from build123d import *

# Parameters (mm, degrees)
SKETCH1_W           = 220
SKETCH1_H           = 40
BOSS_EXTRUDE1_DEPTH = 30
SKETCH2_R           = 10
CUT_EXTRUDE1_DEPTH  = 7
CUT_EXTRUDE2_START  = -30
SKETCH3_R           = 7
CUT_EXTRUDE2_DEPTH  = 23
SKETCH4_W           = 15
SKETCH4_H           = 40
CUT_EXTRUDE3_DEPTH  = 15
CUT_EXTRUDE4_START  = -30
SKETCH5_R           = 2.5
CUT_EXTRUDE4_DEPTH  = 15


with BuildPart() as part:
    # Sketch1 → Boss-Extrude1 (new body)
    with BuildSketch(Plane.XY):
        Rectangle(SKETCH1_W, SKETCH1_H)
    extrude(amount=BOSS_EXTRUDE1_DEPTH)

    # Sketch2 → Cut-Extrude1 (cut)
    with BuildSketch(Plane.XY):
        with Locations((90, 0)):
            Circle(SKETCH2_R)
    extrude(amount=CUT_EXTRUDE1_DEPTH, mode=Mode.SUBTRACT)

    # Sketch3 → Cut-Extrude2 (cut)
    with BuildSketch(Plane(origin=(0, 0, 0), x_dir=(-1, 0, 0), z_dir=(0, 0, -1)).offset(CUT_EXTRUDE2_START)):
        with Locations((-90, 0)):
            Circle(SKETCH3_R)
    extrude(amount=CUT_EXTRUDE2_DEPTH, mode=Mode.SUBTRACT)

    # Sketch4 → Cut-Extrude3 (cut)
    with BuildSketch(Plane(origin=(0, 0, 0), x_dir=(-1, 0, 0), z_dir=(0, 0, -1))):
        with Locations((-22.5, 0)):
            Rectangle(SKETCH4_W, SKETCH4_H)
        with Locations((2.5, 0)):
            Rectangle(SKETCH4_W, SKETCH4_H)
    extrude(amount=-CUT_EXTRUDE3_DEPTH, mode=Mode.SUBTRACT)

    # Sketch5 → Cut-Extrude4 (cut)
    with BuildSketch(Plane(origin=(0, 0, 0), x_dir=(-1, 0, 0), z_dir=(0, 0, -1)).offset(CUT_EXTRUDE4_START)):
        with Locations((-22.5, 10)):
            Circle(SKETCH5_R)
        with Locations((-22.5, -10)):
            Circle(SKETCH5_R)
        with Locations((2.5, -10)):
            Circle(SKETCH5_R)
        with Locations((2.5, 10)):
            Circle(SKETCH5_R)
    extrude(amount=CUT_EXTRUDE4_DEPTH, mode=Mode.SUBTRACT)


solid = part.part
Could you check a few things on this model? Use its own coordinates, in mm. A direction names the side the tool comes from. Give positions to 0.01 mm unless a question says otherwise; leave off trailing zeros. Order: outer loops, then holes, each group sorted by start corner. A loop starts at its lowest first (then second) coordinate and runs counter-clockwise, first axis right, second up. Notation, with made-up numbers: (89.25, -28.75) -> (124.25, -28.75) arc R19 cw to (124.25, 3.25) -> close; hole circle Ø2 at (-9, -39). An arc over 180 degrees is marked (long way). Answer in a Markdown table with one row per item. Add a question column.
Item 1: Please list where these lines run through material, in increasing order: probe 1 along X at (y, z) = (-12, 13.5); probe 2 along Y at (x, z) = (22.5, 24); probe 3 along X at (y, z) = (1.5, 6.75).
Item 2: I'm going to push flat-ended pins straight in: P1, Ø4, axis at x = -23.5, y = 14.5, coming from the -Z side; P2, Ø3, axis at x = -2.5, y = -10, coming from the -Z side; P3, Ø12, axis at x = 23, y = -2.5, coming from the -Z side; P4, Ø6, axis at x = 94.5, y = -4.5, coming from the -Z side. Where does each tip first touch, or does it pass through?
Item 3: Imagine slicing it at A-A (z = 3.5). List the corners of the cut face in (x, y) for me.
Item 4: Imagine slicing it at C-C (x = 22.5). List the corners of the cut face in (y, z) for me.
Item 5: Imagine slicing it at B-B (y = 0). List the corners of the cut face in (x, z) for me.
Item 6: We'd pull the mould along X, two halves only. Please class faces 4 (the flat face through (-61, 0, 0)), 5 (the flat face through (15, 0, 7)), 6 (the flat face through (23, 0, 15)): pulls with the +X half, pulls with the -X half, needs draft (parallel to the pull), parting line crosses it, or undercut.
Item 7: For faces 1 (the flat face through (10, 0, 0)), 2 (the flat face through (-10, 0, 7)), 3 (the cylindrical face through (80, 0, 3)), which set-ups out of +Z, -Z, +X, -X, +Y, -Y let a thin tool reach every point of the face, with its end or its side?
Result:
| question | item | result |
|---|---|---|
| 1 | probe 1 | -110 to -10, 5 to 15, 30 to 110 |
| 1 | probe 2 | -20 to -12.5, -7.5 to 7.5, 12.5 to 20 |
| 1 | probe 3 | -110 to -10, 5 to 15, 30 to 80.11, 99.89 to 110 |
| 2 | P1 | z = 0 |
| 2 | P2 | through |
| 2 | P3 | z = 15 |
| 2 | P4 | z = 7 |
| 3 | outline | (-110, -20) -> (-10, -20) -> (-10, 20) -> (-110, 20) -> close; (5, -20) -> (15, -20) -> (15, 20) -> (5, 20) -> close; (30, -20) -> (110, -20) -> (110, 20) -> (30, 20) -> close; hole circle Ø20 at (90, 0) |
| 4 | outline | (-20, 15) -> (-12.5, 15) -> (-12.5, 30) -> (-20, 30) -> close; (-7.5, 15) -> (7.5, 15) -> (7.5, 30) -> (-7.5, 30) -> close; (12.5, 15) -> (20, 15) -> (20, 30) -> (12.5, 30) -> close |
| 5 | outline | (-110, 0) -> (-10, 0) -> (-10, 15) -> (5, 15) -> (5, 0) -> (15, 0) -> (15, 15) -> (30, 15) -> (30, 0) -> (80, 0) -> (80, 7) -> (83, 7) -> (83, 30) -> (-110, 30) -> close; (97, 7) -> (100, 7) -> (100, 0) -> (110, 0) -> (110, 30) -> (97, 30) -> close |
| 6 | face 4 | needs draft |
| 6 | face 5 | undercut |
| 6 | face 6 | undercut |
| 7 | face 1 | -Z, +X, -X, +Y, -Y |
| 7 | face 2 | -Z, +Y, -Y |
| 7 | face 3 | -Z |
